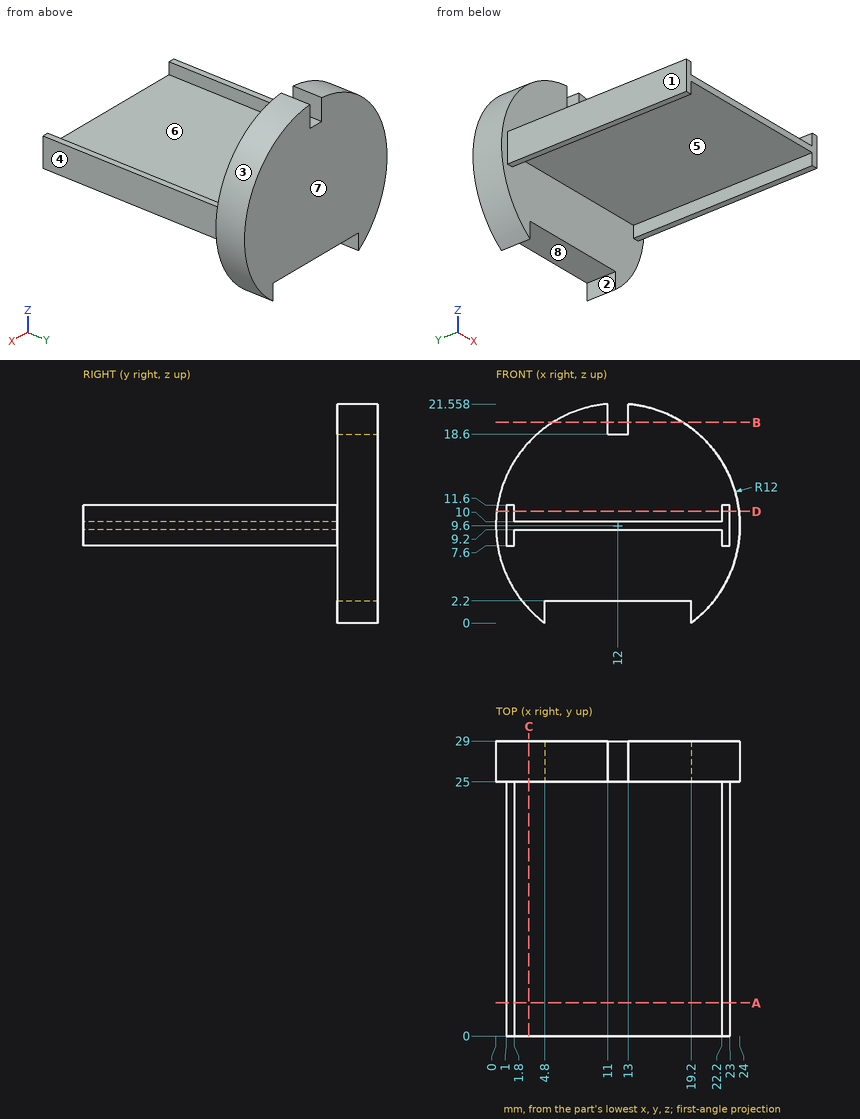
Verification items for this drawing (mm, ordinates from the low corner). A direction names the side the tool comes from. Coordinates: 2 decimals unless noted, no trailing zeros. Order: outer loops, then holes, each group sorted by start corner. A loop starts at its lowest first (then second) coordinate and runs counter-clockwise, first axis right, second up. Notation, with made-up numbers: (12, 23.25) - (34, 23.25) arc R24 cw to (34, 45.25) - close; hole circle Ø1 at (28.25, 32). An arc over 180 degrees is marked (long way). Answer as a JSON object with one key per item and string values. Group by question number.
Item 1: Sectioned sample at B-B, the plane z = 19.75. Record the cut outline in (x, y).
Item 2: Tool access check on the marked faces 4, 5, 6, 7 and 8. Record the directions out of +Z, -Z, +X, -X, +Y, -Y that give a thin tool (end or side, any length) a straight path to the whole face; none if there is none.
Item 3: Sectioned sample at A-A, the plane y = 3.25. Record the cut outline in (x, z).
Item 4: Draft check along X on the marked faces 1, 2 and 3. Enter one of: +X half, -X half, draft (parallel to the pull), parting line (faces both ways), or undercut.
Item 5: Sectioned sample at D-D, the plane z = 11. Record the cut outline in (x, y), and give its area (3 significant figures).
Item 6: Depth check by flat-ended pin: pin 1 Ø1.8 at (y, z) = (28, 1) entering from -X; pin 2 Ø0.9 at (x, y) = (23, 8) entering from -Z; pin 3 Ø4.5 at (y, z) = (17.5, 8.5) entering from +X. Enter the tip coordinate at first touch or a pass-through.
Item 7: Sectioned sample at C-C, the plane x = 3.25. Record the cut outline in (y, z).
Item 8: Scan lines: probe 1 along Z at (x, y) = (12.25, 26.25); probe 2 along X at (y, z) = (6.5, 8.25); probe 3 along Y at (x, z) = (3.5, 2.5). Record each from-to range of solid material in increasing order.
Resolved:
{
 "1": {"outline": "(5.6, 25) - (11, 25) - (11, 29) - (5.6, 29) - close; (13, 25) - (18.4, 25) - (18.4, 29) - (13, 29) - close"},
 "2": {"face 4": "+Z, -Z, +X, -Y", "face 5": "-Z, -Y", "face 6": "+Z, -Y", "face 7": "+Z, -Z, +X, -X, +Y", "face 8": "-Z, +Y, -Y"},
 "3": {"outline": "(1, 7.6) - (1.8, 7.6) - (1.8, 9.2) - (22.2, 9.2) - (22.2, 7.6) - (23, 7.6) - (23, 11.6) - (22.2, 11.6) - (22.2, 10) - (1.8, 10) - (1.8, 11.6) - (1, 11.6) - close"},
 "4": {"face 1": "-X half", "face 2": "undercut", "face 3": "+X half"},
 "5": {"outline": "(0.08, 25) - (1, 25) - (1, 0) - (1.8, 0) - (1.8, 25) - (22.2, 25) - (22.2, 0) - (23, 0) - (23, 25) - (23.92, 25) - (23.92, 29) - (0.08, 29) - close", "area": "135 mm^2"},
 "6": {"pin 1": "x = 2.8", "pin 2": "z = 7.6", "pin 3": "x = 23"},
 "7": {"outline": "(0, 9.2) - (25, 9.2) - (25, 1.39) - (29, 1.39) - (29, 17.81) - (25, 17.81) - (25, 10) - (0, 10) - close"},
 "8": {"probe 1": "2.2 to 18.6", "probe 2": "1 to 1.8, 22.2 to 23", "probe 3": "25 to 29"}
}
